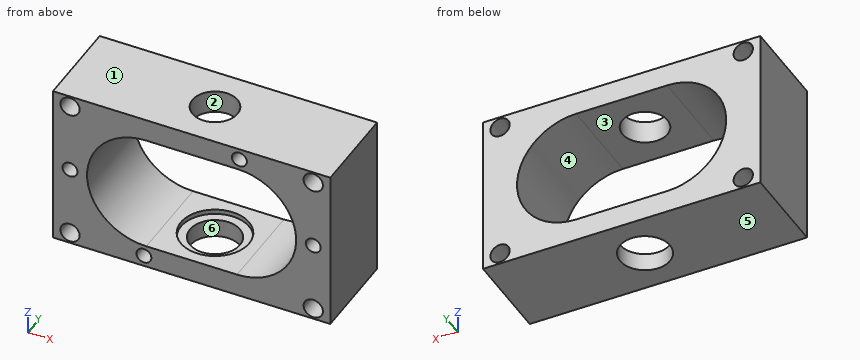
from build123d import *

# Parameters (mm, degrees)
F0_W     = 122
F0_H     = 72
F1_DEPTH = 40
F2_D     = 6.6
F2_DEPTH = 15
F2_TIP   = 1.9828400428
F3_D     = 8.5
F5_D     = 19.84248
F5_DEPTH = 15
F5_TIP   = 5.9612824079
F6_R     = 11
F7_DEPTH = 25
F8_R     = 15
F9_DEPTH = 2.1


with BuildPart() as f1:
    # F0 (on Front) → F1 (new body)
    with BuildSketch(Plane.XZ):
        Rectangle(F0_W, F0_H)
        with BuildLine():
            ThreePointArc((-19.9292801285, -25.999903821), (-45.9999759552, -0.0353599684), (-20, 26))
            Line((-20, 26), (20, 26))
            ThreePointArc((20, 26), (46, 0), (20, -26))
            Line((20, -26), (-19.9292801285, -25.999903821))
        make_face(mode=Mode.SUBTRACT)
    extrude(amount=-F1_DEPTH)

    # F2
    with Locations(Plane.XZ):
        with Locations((21, 31), (53.5, 0), (-21, -31), (-53.5, 0)):
            Hole(F2_D / 2, depth=F2_DEPTH)
            with Locations((0, 0, -(F2_DEPTH + F2_TIP / 2))):  # 118° drill point
                Cone(0, F2_D / 2, F2_TIP, mode=Mode.SUBTRACT)

    # F3 (through all)
    with Locations(Plane.XZ):
        with Locations((-53.5, 31), (-53.5, -31), (53.5, 31), (53.5, -31)):
            Hole(F3_D / 2)

    # F5
    with Locations(Plane.XY.offset(36)):
        with Locations((0, 20)):
            Hole(F5_D / 2, depth=F5_DEPTH)
            with Locations((0, 0, -(F5_DEPTH + F5_TIP / 2))):  # 118° drill point
                Cone(0, F5_D / 2, F5_TIP, mode=Mode.SUBTRACT)

    # F6 (on face) → F7 (cut)
    with BuildSketch(Plane(origin=(0, 0, -36), x_dir=(1, 0, 0), z_dir=(0, 0, -1))):
        with Locations((0, -20)):
            Circle(F6_R)
    extrude(amount=-F7_DEPTH, mode=Mode.SUBTRACT)

    # F8 (on face) → F9 (cut)
    with BuildSketch(Plane(origin=(-6.2627e-05, 0, -25.9999518252), x_dir=(1, 0, -2.4087e-06), z_dir=(2.4087e-06, 0, 1))):
        with Locations((6.2627e-05, 20)):
            Circle(F8_R)
    extrude(amount=-F9_DEPTH, mode=Mode.SUBTRACT)


solid = f1.part
Can you work these out from the model? Positions are in its coordinate system, mm. Face numbers are marked on the shaded views. A direction names the side the tool comes from. Give positions to 0.01 mm unless a question says otherwise; leave off trailing zeros. Loops run counter-clockwise (first coordinate to the right, second up) from the corner with the lowest first, then second, coordinate; pieces in that order, holes last. Notation, with made-up numbers: (69, -28) - (88, -28) arc R19 cw to (88, -15) - close; hole circle Ø7 at (57, -2). An arc over 180 degrees is marked (long way). Return JSON: item names as keys, results as strings.
1. We'd pull the mould along Z, two halves only. Please class the marked faces 1, 2 and 3: +Z half, -Z half, draft (parallel to the pull), parting line (faces both ways), or undercut.
Output values:
{"face 1": "+Z half", "face 2": "draft", "face 3": "undercut"}
2. For the marked faces 4, 5 and 6, which set-ups out of +Z, -Z, +X, -X, +Y, -Y let a thin tool reach every point of the face, with its end or its side?
Output values:
{"face 4": "+Y, -Y", "face 5": "-Z, +X, -X, +Y, -Y", "face 6": "-Z"}
3. If I drill on line 1 (Z direction, x = -53.5, y = 26); line 2 (Z direction, x = -16, y = 9); line 3 (Z direction, x = 0, y = 34), over which ranges is the centre line in solid material (lowest first)?
Output values:
{"line 1": "z = -36 to -35.25, -26.75 to 26.75, 35.25 to 36", "line 2": "z = -36 to -26, 26 to 36", "line 3": "z = -36 to -28.1, 26 to 36"}
4. I want a section at A-A on y = 20. Please give me the cut outline in (x, z).
Output values:
{"outline": "(-61, -36) - (-11, -36) - (-11, -28.1) - (-15, -28.1) - (-15, -26) - (-19.93, -26) arc R26 cw to (-20, 26) - (-9.92, 26) - (-9.92, 36) - (-61, 36) - close; (9.92, 26) - (20, 26) arc R26 cw to (20, -26) - (15, -26) - (15, -28.1) - (11, -28.1) - (11, -36) - (61, -36) - (61, 36) - (9.92, 36) - close; hole circle Ø8.5 at (-53.5, -31); hole circle Ø8.5 at (-53.5, 31); hole circle Ø8.5 at (53.5, -31); hole circle Ø8.5 at (53.5, 31)"}
5. I want a section at D-D on y = 27. Please give me the cut outline in (x, z).
Output values:
{"outline": "(-61, -36) - (-8.49, -36) - (-8.49, -28.1) - (-13.27, -28.1) - (-13.27, -26) - (-19.93, -26) arc R26 cw to (-20, 26) - (-7.03, 26) - (-7.03, 36) - (-61, 36) - close; (7.03, 26) - (20, 26) arc R26 cw to (20, -26) - (13.27, -26) - (13.27, -28.1) - (8.49, -28.1) - (8.49, -36) - (61, -36) - (61, 36) - (7.03, 36) - close; hole circle Ø8.5 at (-53.5, -31); hole circle Ø8.5 at (-53.5, 31); hole circle Ø8.5 at (53.5, -31); hole circle Ø8.5 at (53.5, 31)"}
6. I'm going to push flat-ended pins straight in: pin 1 Ø7.5 at (x, z) = (-53.5, -31) entering from +Y; pin 2 Ø4 at (x, z) = (-53.5, 0) entering from -Y. Where does each tip first touch, or does it pass through?
Output values:
{"pin 1": "passes through", "pin 2": "stops at y = 15.78"}
7. I want a section at B-B on z = -18. Please give me the cut outline in (x, y), and give its area (3 significant figures).
Output values:
{"outline": "(-61, 0) - (-38.76, 0) - (-38.76, 40) - (-61, 40) - close; (38.76, 0) - (61, 0) - (61, 40) - (38.76, 40) - close", "area": "1,780 mm²"}
8. I want a section at C-C on x = 0. Give the number of separate pieces and of enclosed holes in the cut face, and give its area (3 significant figures).
Output values:
{"separate pieces": "4", "enclosed holes": "0", "area": "365 mm²"}
